from build123d import *

# Parameters (mm, degrees)
SKETCH2_R           = 1.3
BOSS_EXTRUDE1_DEPTH = 3
SKETCH3_W           = 6.35
SKETCH3_H           = 3
BOSS_EXTRUDE2_DEPTH = 3
LPATTERN1_COUNT     = 4
LPATTERN1_PITCH     = 12.7


with BuildPart() as part:
    # Sketch2 → Boss-Extrude1 (new body)
    with BuildSketch(Plane.XY):
        with BuildLine():
            Line((0, 6), (-27.965559662, 7.439126041))
            ThreePointArc((-27.965559662, 7.439126041), (-32.639, 3), (-27.965559662, -1.439126041))
            Line((-27.965559662, -1.439126041), (0, 0))
            Line((0, 0), (50.8, 0))
            Line((50.8, 0), (50.8, 6))
            Line((50.8, 6), (0, 6))
        make_face()
        with Locations((-28.194, 3)):
            Circle(SKETCH2_R, mode=Mode.SUBTRACT)
    extrude(amount=BOSS_EXTRUDE1_DEPTH)

    # Sketch3 → Boss-Extrude2 (add)
    with BuildSketch(Plane.XZ):
        with Locations((6.35, 1.5)):
            Rectangle(SKETCH3_W, SKETCH3_H)
    boss_extrude2 = extrude(amount=BOSS_EXTRUDE2_DEPTH)

    # LPattern1: Boss-Extrude2 ×4
    with Locations(*[(i * LPATTERN1_PITCH, 0, 0) for i in range(1, LPATTERN1_COUNT)]):
        add(boss_extrude2)


solid = part.part
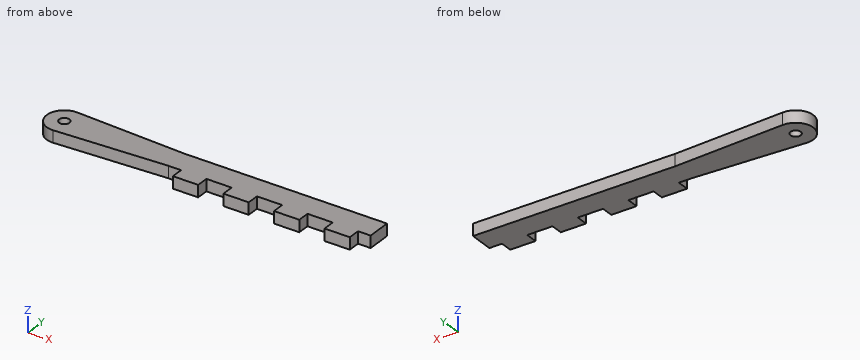
Read the model definition and answer for the solid it produces. Units are mm, in the model's axes. Give positions to 0.01 mm unless a question says otherwise; leave off trailing zeros. Loops run counter-clockwise (first coordinate to the right, second up) from the corner with the lowest first, then second, coordinate; pieces in that order, holes last. Notation, with made-up numbers: (77.25, -32.5) - (121.25, -32.5) arc R13 ccw to (121.25, -15.5) - close; hole circle Ø11 at (58, -27). An arc over 180 degrees is marked (long way). Answer as CSV lines item,"result". Start each with the question number.
1) Straight lines are drawn through the part: L1, parallel to Y at x = -28, z = 1.55; L2, parallel to Y at x = 39, z = 1.45; L3, parallel to Y at x = 18, z = 2.7. For each, find the intervals that lie inside material, in ascending order. Write a range as from..to.
2) Find section D-D (x = 21). Write down the section's boundary in (y, z), then the cut area to 3 significant figures.
3) Find section A-A (y = 3). Write down the section's boundary in (x, z).
4) Find section B-B (z = 0.85). Write down the section's boundary in (x, y) (3 decimals), then the cut area to 3 significant figures.
5) Find section C-C (x = 36.5). Write down the section's boundary in (y, z).
6) Each of these flat-tipped pins is pushed along its axis until it touches: pin 1 Ø0.9 at (x, z) = (50, 1.5) entering from -Y; pin 2 Ø1.5 at (y, z) = (-1, 1) entering from -X; pin 3 Ø0.9 at (y, z) = (-1, 1.5) entering from +X (3 decimals); pin 4 Ø2 at (x, y) = (-28.194, 3) entering from -Z. Where does it stop, or does it pass through?
Findings below:
1,L1,"-1.44..1.71, 4.29..7.44"
1,L2,"0..6"
1,L3,"-3..6"
2,outline,"(-3, 0) - (6, 0) - (6, 3) - (-3, 3) - close"
2,area,"27.0 mm^2"
3,outline,"(-32.64, 0) - (-29.49, 0) - (-29.49, 3) - (-32.64, 3) - close; (-26.89, 0) - (50.8, 0) - (50.8, 3) - (-26.89, 3) - close"
4,outline,"(-27.966, -1.439) - (0, 0) - (3.175, 0) - (3.175, -3) - (9.525, -3) - (9.525, 0) - (15.875, 0) - (15.875, -3) - (22.225, -3) - (22.225, 0) - (28.575, 0) - (28.575, -3) - (34.925, -3) - (34.925, 0) - (41.275, 0) - (41.275, -3) - (47.625, -3) - (47.625, 0) - (50.8, 0) - (50.8, 6) - (0, 6) - (-27.966, 7.439) arc R4.445 ccw (long way) to start; hole circle Ø2.6 at (-28.194, 3)"
4,area,"617 mm^2"
5,outline,"(0, 0) - (6, 0) - (6, 3) - (0, 3) - close"
6,pin 1,"y = 0"
6,pin 2,"x = -31.23"
6,pin 3,"x = 47.625"
6,pin 4,"through"
